```python
from build123d import *

# Parameters (mm, degrees)
SKETCH1_R           = 10
SKETCH1_R_2         = 7.5
BOSS_EXTRUDE1_DEPTH = 1
SKETCH1_3_R         = 7.5
SKETCH1_3_R_2       = 5
BOSS_EXTRUDE2_DEPTH = 10
FILLET1_R           = 1


with BuildPart() as part:
    # Sketch1 → Boss-Extrude1 (new body)
    with BuildSketch(Plane(origin=(0, 0, 0), x_dir=(-1, 0, 0), z_dir=(0, 1, 0))):
        with Locations(Location((0, 0, 0), (0, 0, 90))):
            Circle(SKETCH1_R)
        with Locations(Location((0, 0, 0), (0, 0, 90))):
            Circle(SKETCH1_R_2, mode=Mode.SUBTRACT)
    extrude(amount=BOSS_EXTRUDE1_DEPTH)

    # Sketch1_3 → Boss-Extrude2 (add)
    with BuildSketch(Plane(origin=(0, 0, 0), x_dir=(-1, 0, 0), z_dir=(0, 1, 0))):
        with Locations(Location((0, 0, 0), (0, 0, 90))):
            Circle(SKETCH1_3_R)
        with Locations(Location((0, 0, 0), (0, 0, 90))):
            Circle(SKETCH1_3_R_2, mode=Mode.SUBTRACT)
    extrude(amount=BOSS_EXTRUDE2_DEPTH)

    # Fillet1
    fillet1_edges = [part.edges().sort_by_distance(p)[0] for p in [
        (0, 1, -7.5),
    ]]
    fillet(fillet1_edges, radius=FILLET1_R)


solid = part.part
```
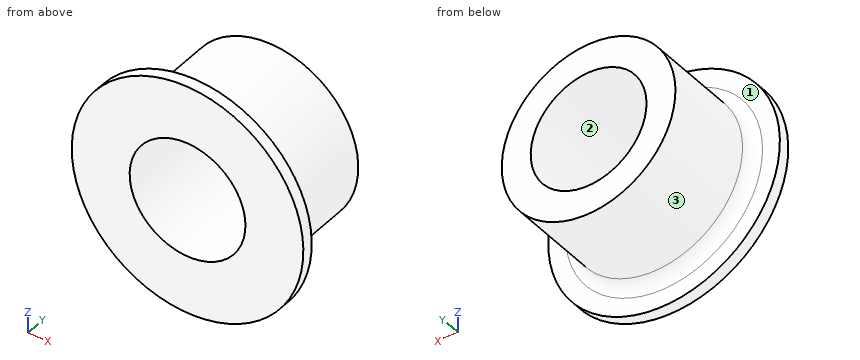
Input: part model. Units: mm. Frame: model coordinates. Face numbers are marked on the shaded views. Round coordinates to 2 decimals unless told otherwise and drop trailing zeros. Loops run counter-clockwise (first coordinate to the right, second up) from the corner with the lowest first, then second, coordinate; pieces in that order, holes last.
1) Section query D-D on x = 8.75. Return the cut outline in (y, z), plus the area to 3 significant figures.
Ans:
outline: (0, -4.84) - (1, -4.84) - (1, 4.84) - (0, 4.84) - close
area: 9.68 mm2
2) Material intervals for line 1 (X direction, y = 3.25, z = 0); line 2 (Z direction, x = 2.5, y = 9.5); line 3 (X direction, y = 0.5, z = 3.25), sorted ascending.
Ans:
line 1: x = -7.5 to -5, 5 to 7.5
line 2: z = -7.07 to -4.33, 4.33 to 7.07
line 3: x = -9.46 to -3.8, 3.8 to 9.46
3) Section query A-A on x = 0. Return the cut outline in (y, z), plus the area to 3 significant figures.
Ans:
outline: (0, -10) - (1, -10) - (1, -8.5) arc R1 cw to (2, -7.5) - (10, -7.5) - (10, -5) - (0, -5) - close; (0, 5) - (10, 5) - (10, 7.5) - (2, 7.5) arc R1 cw to (1, 8.5) - (1, 10) - (0, 10) - close
area: 55.4 mm2
4) Section query C-C on y = 4. Return the cut outline in (x, z), plus the area to 3 significant figures.
Ans:
outline: circle Ø15 at (0, 0); hole circle Ø10 at (0, 0)
area: 98.2 mm2
5) Pull-direction query (X, two-part tool) for the marked faces 1, 2 and 3; classes: released by +X, released by -X, zero draft, split by the parting line, or undercut.
Ans:
face 1: zero draft
face 2: undercut
face 3: split by the parting line
6) Pin query (flat end, axial travel): pin 1 (1.5 mm diameter, centred on y = 7, z = -0.5, fed in from +X); pin 2 (3 mm diameter, centred on x = -5.5, z = -6.5, fed in from +Y); pin 3 (2 mm diameter, centred on x = -3.5, y = 5, fed in from +Z); pin 4 (2 mm diameter, centred on y = 5, z = -5.5, fed in from -X). Return the tip coordinate at first contact, or that it passes through.
Ans:
pin 1: stops at x = 7.5
pin 2: stops at y = 10
pin 3: stops at z = 7.07
pin 4: stops at x = -6
7) Section query B-B on z = 0. Return the cut outline in (x, y).
Ans:
outline: (-10, 0) - (-5, 0) - (-5, 10) - (-7.5, 10) - (-7.5, 2) arc R1 cw to (-8.5, 1) - (-10, 1) - close; (5, 0) - (10, 0) - (10, 1) - (8.5, 1) arc R1 cw to (7.5, 2) - (7.5, 10) - (5, 10) - close
